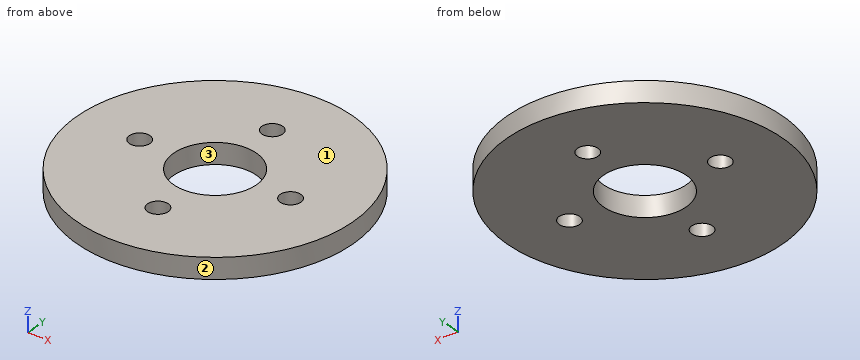
from build123d import *

# Parameters (mm, degrees)
SKETCH_1_R          = 20
SKETCH_1_R_2        = 1.5
EXTRUDE_1_DEPTH     = 3
SKETCH_2_R          = 6
CUT_EXTRUDE_1_DEPTH = 29.442925307


with BuildPart() as part:
    # 草图1 → 凸台-拉伸1 (new body)
    with BuildSketch(Plane.XY):
        Circle(SKETCH_1_R)
        with Locations((0, 11)):
            Circle(SKETCH_1_R_2, mode=Mode.SUBTRACT)
        with Locations((11, 0)):
            Circle(SKETCH_1_R_2, mode=Mode.SUBTRACT)
        with Locations((0, -11)):
            Circle(SKETCH_1_R_2, mode=Mode.SUBTRACT)
        with Locations((-11, 0)):
            Circle(SKETCH_1_R_2, mode=Mode.SUBTRACT)
    extrude(amount=EXTRUDE_1_DEPTH)

    # 草图2 → 切除-拉伸1 (cut, through all)
    with BuildSketch(Plane.XY.offset(3)):
        Circle(SKETCH_2_R)
    extrude(amount=-CUT_EXTRUDE_1_DEPTH, mode=Mode.SUBTRACT)


solid = part.part
CAD build for the part. Positions are in the model's coordinates, mm. Face numbers are marked on the shaded views. Round coordinates to 2 decimals unless told otherwise and drop trailing zeros. Write each loop counter-clockwise with the first axis right and the second up, starting at its lowest first coordinate (ties: lowest second). Pieces come first, ordered by that corner, then holes.
(1) Drop a flat-ended pin along its axis: P1, Ø1, axis at x = 6.5, z = 1, coming from the -Y side. Give the stop position or say it passes through.
(2) Slice it at D-D, the plane y = 11. Write the cut outline in (x, z), and give its area (3 significant figures).
(3) Slice it at A-A, the plane x = 0. Write the cut outline in (y, z), and give its area (3 significant figures).
(4) Slice it at C-C, the plane z = 1.25. Write the cut outline in (x, y).
(5) Mould opens along X. For the marked faces 1, 2 and 3 say: pulls with the +X half, pulls with the -X half, needs draft (parallel to the pull), parting line crosses it, or undercut.
(6) Probe line 1 along Y through (x, z) = (0, 0.85); line 2 along Y through (x, z) = (-12, 0.1); line 3 along Y through (x, z) = (11, 0.85). List the from-to ranges inside material, lowest first.
From the geometry:
1. P1: stops at y = -19.08
2. outline: (-16.7, 0) - (-1.5, 0) - (-1.5, 3) - (-16.7, 3) - close; (1.5, 0) - (16.7, 0) - (16.7, 3) - (1.5, 3) - close
2. area: 91.2 mm2
3. outline: (-20, 0) - (-12.5, 0) - (-12.5, 3) - (-20, 3) - close; (-9.5, 0) - (-6, 0) - (-6, 3) - (-9.5, 3) - close; (6, 0) - (9.5, 0) - (9.5, 3) - (6, 3) - close; (12.5, 0) - (20, 0) - (20, 3) - (12.5, 3) - close
3. area: 66.0 mm2
4. outline: circle Ø40 at (0, 0); hole circle Ø3 at (-11, 0); hole circle Ø12 at (0, 0); hole circle Ø3 at (0, -11); hole circle Ø3 at (0, 11); hole circle Ø3 at (11, 0)
5. face 1: needs draft
5. face 2: parting line crosses it
5. face 3: undercut
6. line 1: y = -20 to -12.5, -9.5 to -6, 6 to 9.5, 12.5 to 20
6. line 2: y = -16 to -1.12, 1.12 to 16
6. line 3: y = -16.7 to -1.5, 1.5 to 16.7
